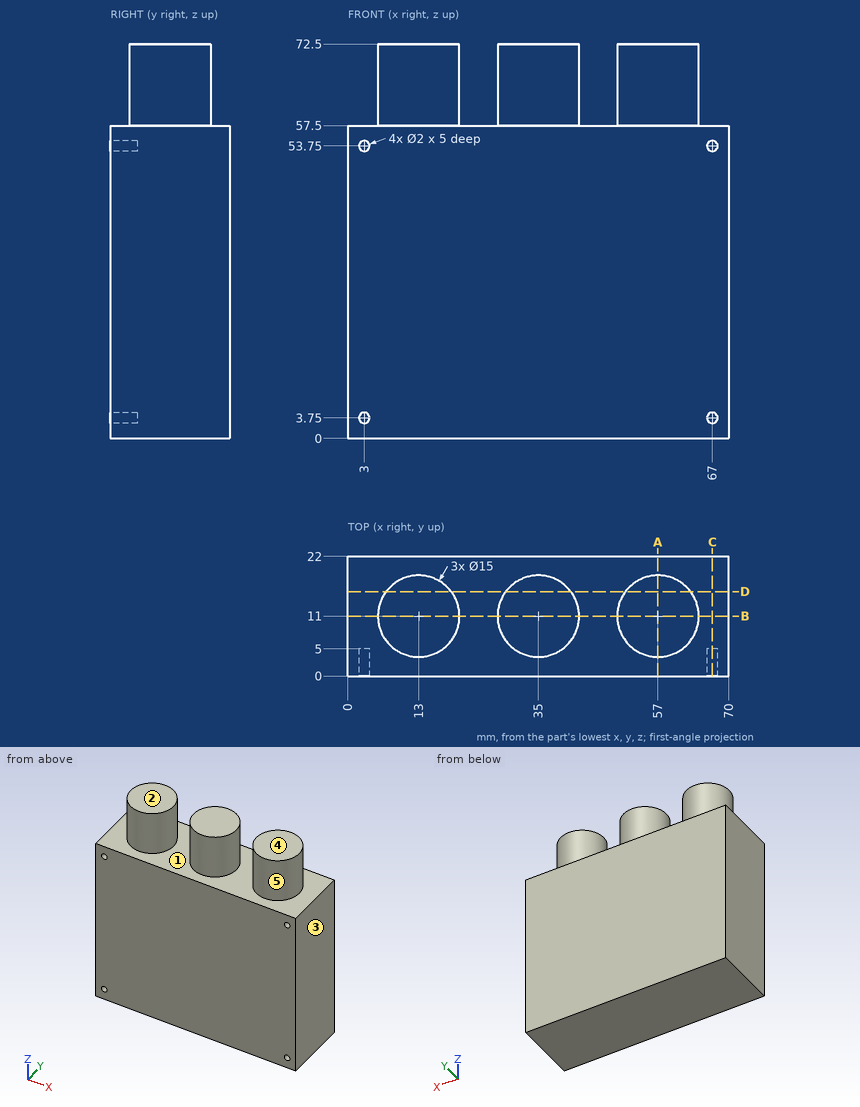
Source: three-view drawing plus pictorial views. Frame: mm from the lowest corner of the part. A direction names the side the tool comes from. Coordinates: 2 decimals unless noted, no trailing zeros. Write each loop counter-clockwise with the first axis right and the second up, starting at its lowest first coordinate (ties: lowest second). Pieces come first, ordered by that corner, then holes. Notation, with made-up numbers: (63, 69) - (99, 69) arc R19 cw to (99, 87) - close; hole circle Ø9 at (41, -23.5). An arc over 180 degrees is marked (long way). Answer as a JSON object with one key per item and string values.
Q1. Set-up query: the marked faces 1 and 2. Return all of +Z, -Z, +X, -X, +Y, -Y with unobstructed straight access to the full face (end or side cutting, diameter ignored); none if empty.
Ans:
{"face 1": "+Z", "face 2": "+Z, +X, -X, +Y, -Y"}
Q2. Section query B-B, the plane y = 11. Output: boundary loops of the cut face in (x, z).
Ans:
{"outline": "(0, 0) - (70, 0) - (70, 57.5) - (64.5, 57.5) - (64.5, 72.5) - (49.5, 72.5) - (49.5, 57.5) - (42.5, 57.5) - (42.5, 72.5) - (27.5, 72.5) - (27.5, 57.5) - (20.5, 57.5) - (20.5, 72.5) - (5.5, 72.5) - (5.5, 57.5) - (0, 57.5) - close"}
Q3. First-contact query: pin 1 Ø0.6 at (x, z) = (3.5, 53.5) entering from -Y; pin 2 Ø4 at (x, y) = (51, 3.5) entering from +Z. Flat tips, straight axial feed; report the tip coordinate or a pass-through.
Ans:
{"pin 1": "stops at y = 5", "pin 2": "stops at z = 57.5"}
Q4. Draft query along X for the marked faces 3, 4 and 5. Return one class per face: released by +X, released by -X, zero draft, split by the parting line, or undercut.
Ans:
{"face 3": "released by +X", "face 4": "zero draft", "face 5": "undercut"}
Q5. Section query A-A, the plane x = 57. Output: boundary loops of the cut face in (y, z).
Ans:
{"outline": "(0, 0) - (22, 0) - (22, 57.5) - (18.5, 57.5) - (18.5, 72.5) - (3.5, 72.5) - (3.5, 57.5) - (0, 57.5) - close"}
Q6. Section query D-D, the plane y = 15.5. Output: boundary loops of the cut face in (x, z).
Ans:
{"outline": "(0, 0) - (70, 0) - (70, 57.5) - (63, 57.5) - (63, 72.5) - (51, 72.5) - (51, 57.5) - (41, 57.5) - (41, 72.5) - (29, 72.5) - (29, 57.5) - (19, 57.5) - (19, 72.5) - (7, 72.5) - (7, 57.5) - (0, 57.5) - close"}
Q7. Material intervals for line 1 (X direction, y = 1.1, z = 53.75); line 2 (Z direction, x = 67, y = 3.1); line 3 (X direction, y = 7.5, z = 59), sorted ascending. Write a range as [from, to].
Ans:
{"line 1": "x = [0, 2], [4, 66], [68, 70]", "line 2": "z = [0, 2.75], [4.75, 52.75], [54.75, 57.5]", "line 3": "x = [6.37, 19.63], [28.37, 41.63], [50.37, 63.63]"}
Q8. Section query C-C, the plane x = 67. Output: boundary loops of the cut face in (y, z), plus the area to 4 significant figures.
Ans:
{"outline": "(0, 0) - (22, 0) - (22, 57.5) - (0, 57.5) - (0, 54.75) - (5, 54.75) - (5, 52.75) - (0, 52.75) - (0, 4.75) - (5, 4.75) - (5, 2.75) - (0, 2.75) - close", "area": "1,245 mm2"}
